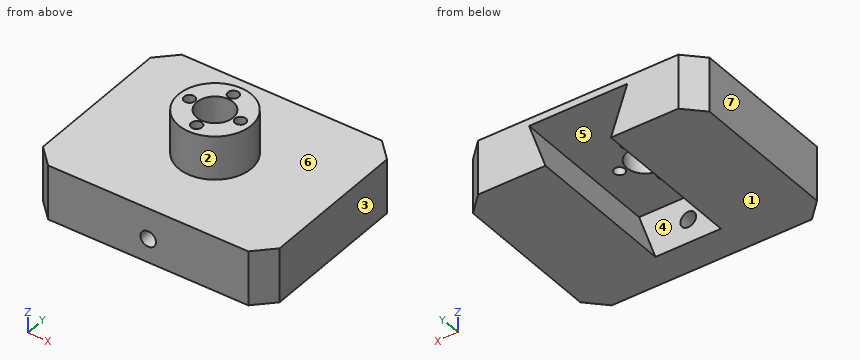
Autodesk Inventor part; units mm, degrees
ref_plane "YZ Plane" through (0, 0, 0) normal (1, 0, 0) x (0, 1, 0)
ref_plane "XZ Plane" through (0, 0, 0) normal (0, 1, 0) x (-1, 0, 0)
ref_plane "XY Plane" through (0, 0, 0) normal (0, 0, 1) x (1, 0, 0)
sketch "Skizze1" plane through (0, 0, 0) normal (0, 0, 1) x (1, 0, 0)
  line L0 (-32.5, 25.5) -> (32.5, 25.5)
  line L1 (32.5, 25.5) -> (32.5, -25.5)
  line L2 (32.5, -25.5) -> (-32.5, -25.5)
  line L3 (-32.5, -25.5) -> (-32.5, 25.5)
  line L4 (0, -35.7) -> (0, 35.7)
  line L5 (-45.5, 0) -> (45.5, 0)
  point P0 (0, 0)
  point P1 (0, 25.5)
  point P2 (32.5, 0)
  dimension "d0" = 51
  dimension "d1" = 65
extrude "Extrusion1" add sketch "Skizze1" along normal blind 15
sketch "Skizze2" plane through (-32.5, -25.5, 0) normal (0, -1, 0) x (1, 0, 0)
  line L0 (23.5, 0) -> (41.5, 0)
  line L1 (41.5, 0) -> (46, 13)
  line L2 (46, 13) -> (19, 13)
  line L3 (19, 13) -> (23.5, 0)
  line L4 (0, 0) -> (65, 0)
  line L5 (0, 15) -> (65, 15) construction
  circle A0 centre (32.5, 6.5) radius 2.15
  line L6 (32.5, 0) -> (32.5, 13) construction
  point P0 (32.5, 0)
  point P1 (32.5, 6.5)
  dimension "d4" = 18
  dimension "d5" = 27
  dimension "d6" = 13
  dimension "d20" = 4.3
extrude "Extrusion2" cut sketch "Skizze2" against normal through all contours L3 L2 L1 L0 | A0
extrude "Extrusion5" add sketch "Skizze2" against normal blind 9
chamfer "Fase1" distance 5 angle 45 4 edges at (-32.5, 25.5, 7.5) (32.5, 25.5, 7.5) (32.5, -25.5, 7.5) (-32.5, -25.5, 7.5)
sketch "Skizze3" plane through (0, 0, 15) normal (0, 0, 1) x (1, 0, 0)
  circle A0 centre (0, 0) radius 10
  dimension "d12" = 20
extrude "Extrusion3" add sketch "Skizze3" along normal blind 12
sketch "Skizze4" plane through (0, 0, 27) normal (0, 0, 1) x (1, 0, 0)
  circle A0 centre (0, 0) radius 5
  dimension "d15" = 10
extrude "Extrusion4" cut sketch "Skizze4" against normal through all
sketch "Skizze5" plane through (0, 0, 27) normal (0, 0, 1) x (1, 0, 0)
  circle A0 centre (7, 0) radius 1.5
  line L0 (-45.5, 0) -> (45.5, 0)
  circle A1 centre (0, 0) radius 5
  circle A2 centre (0, 0) radius 10
  circle A3 centre (0, 7) radius 1.5
  circle A4 centre (-7, 0) radius 1.5
  circle A5 centre (0, -7) radius 1.5
  dimension "d21" = 3
  dimension "d22" = 7
  dimension "d25" = 360
extrude "Extrusion6" cut sketch "Skizze5" against normal through all contours L0 A0 | A0 L0 | A4 L0 | L0 A4 | A3 | A5
sketch "Skizze6" plane through (0, 0, 27) normal (0, 0, 1) x (1, 0, 0)
  line L0 (15.25, -15.25) -> (-15.25, -15.25)
  line L1 (-15.25, -15.25) -> (-15.25, 15.25)
  line L2 (-15.25, 15.25) -> (15.25, 15.25)
  line L3 (15.25, 15.25) -> (15.25, -15.25)
  line L4 (15.25, -15.25) -> (-15.25, 15.25) construction
  line L5 (-15.25, -15.25) -> (15.25, 15.25) construction
  circle A0 centre (15.25, 15.25) radius 2
  circle A1 centre (-15.25, 15.25) radius 2
  circle A2 centre (-15.25, -15.25) radius 2
  circle A3 centre (15.25, -15.25) radius 2
  point P0 (0, 0)
  dimension "d29" = 30.5
  dimension "d30" = 4
extrude "Extrusion7" [suppressed]
properties part number "_3D-Druck"
CAD build for the part. Positions are in the model's coordinates, mm. Face numbers are marked on the shaded views. A direction names the side the tool comes from. Give positions to 0.01 mm unless a question says otherwise; leave off trailing zeros. Write each loop counter-clockwise with the first axis right and the second up, starting at its lowest first coordinate (ties: lowest second). Pieces come first, ordered by that corner, then holes. Notation, with made-up numbers: (11, 8) - (63, 8) arc R18 ccw to (63, 12) - close; hole circle Ø2 at (23, 26.25). An arc over 180 degrees is marked (long way). Put each result on its own line as item: value.
(1) Tool access for the marked faces 5, 6 and 7: list every direction of +Z, -Z, +X, -X, +Y, -Y with a clear straight run to the whole face (end or side of a thin tool).
Working result:
face 5: +Y
face 6: +Z
face 7: +Z, -Z, -X, +Y, -Y
(2) Saw through at D-D (y = 17). List the corners of the cut face in (x, z).
Working result:
outline: (-32.5, 0) - (-9, 0) - (-13.5, 13) - (13.5, 13) - (9, 0) - (32.5, 0) - (32.5, 15) - (-32.5, 15) - close
(3) Saw through at B-B (y = 0). List the corners of the cut face in (x, z), then the cut area to 4 significant figures.
Working result:
outline: (-32.5, 0) - (-9, 0) - (-13.5, 13) - (-8.5, 13) - (-8.5, 27) - (-10, 27) - (-10, 15) - (-32.5, 15) - close; (-5.5, 13) - (-5, 13) - (-5, 27) - (-5.5, 27) - close; (5, 13) - (5.5, 13) - (5.5, 27) - (5, 27) - close; (8.5, 13) - (13.5, 13) - (9, 0) - (32.5, 0) - (32.5, 15) - (10, 15) - (10, 27) - (8.5, 27) - close
area: 698.5 mm^2
(4) Wall check: L1, parallel to Y at x = 0, z = 20.75; L2, parallel to Z at x = -23, y = 10.5; L3, parallel to Y at x = -7, z = 21.75. Give the ranges that are in metal, low to high.
Working result:
L1: -10 to -8.5, -5.5 to -5, 5 to 5.5, 8.5 to 10
L2: 0 to 15
L3: -7.14 to -1.5, 1.5 to 7.14
(5) Pull direction X, two halves, no side cores. Call the marked faces 1, 2, 3 and 4: released by +X, released by -X, zero draft, split by the parting line, or undercut.
Working result:
face 1: zero draft
face 2: split by the parting line
face 3: released by +X
face 4: undercut
(6) Saw through at C-C (z = 6.5). List the corners of the cut face in (x, y), then the cut area to 3 significant figures.
Working result:
outline: (-32.5, -20.5) - (-27.5, -25.5) - (-2.15, -25.5) - (-2.15, -16.5) - (-11.25, -16.5) - (-11.25, 25.5) - (-27.5, 25.5) - (-32.5, 20.5) - close; (2.15, -25.5) - (27.5, -25.5) - (32.5, -20.5) - (32.5, 20.5) - (27.5, 25.5) - (11.25, 25.5) - (11.25, -16.5) - (2.15, -16.5) - close
area: 2,280 mm^2
(7) Drop flat-ended pins along their axis: pin 1 Ø1.5 at (x, y) = (22, 15.5) entering from +Z; pin 2 Ø3.5 at (x, y) = (7, 0) entering from -Z; pin 3 Ø6 at (y, z) = (1.5, 19) entering from -X. Give the stop position or say it passes through.
Working result:
pin 1: z = 15
pin 2: z = 13
pin 3: x = -10
(8) Saw through at A-A (x = 0). List the corners of the cut face in (y, z).
Working result:
outline: (-25.5, 0) - (-16.5, 0) - (-16.5, 4.35) - (-25.5, 4.35) - close; (-25.5, 8.65) - (-16.5, 8.65) - (-16.5, 13) - (-8.5, 13) - (-8.5, 27) - (-10, 27) - (-10, 15) - (-25.5, 15) - close; (-5.5, 13) - (-5, 13) - (-5, 27) - (-5.5, 27) - close; (5, 13) - (5.5, 13) - (5.5, 27) - (5, 27) - close; (8.5, 13) - (25.5, 13) - (25.5, 15) - (10, 15) - (10, 27) - (8.5, 27) - close
